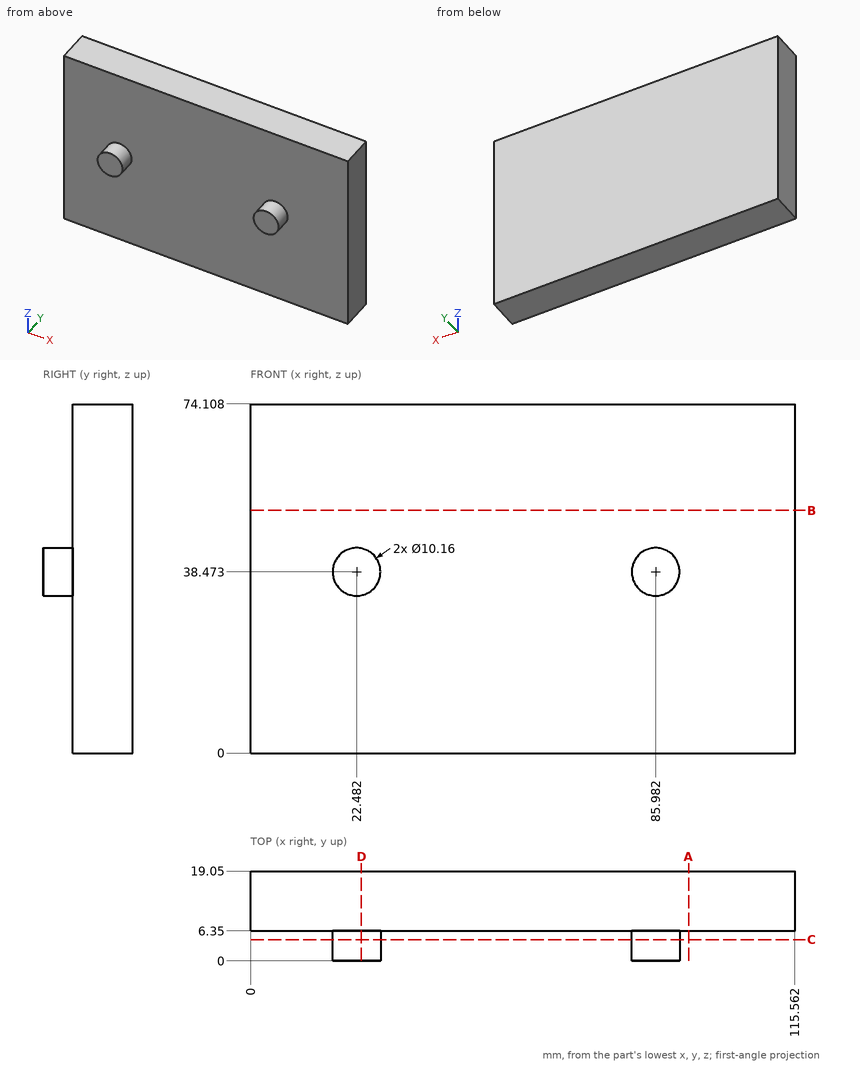
Part print with two shaded views. Sizes in mm from the minimum x, y, z corner. Coordinates: 2 decimals unless noted, no trailing zeros. Write each loop counter-clockwise with the first axis right and the second up, starting at its lowest first coordinate (ties: lowest second). Pieces come first, ordered by that corner, then holes. Notation, with made-up numbers: (63, -26.5) -> (108, -26.5) arc R17 ccw to (108, -12.5) -> close; hole circle Ø5 at (76.5, 5.5). An arc over 180 degrees is marked (long way). Return JSON: item names as keys, results as strings. Group by question number.
Q1. Cut at D-D, the plane x = 23.5. Give the cut face in (y, z), then the cut area to 3 significant figures.
Q2. Drill centre lines: line 1 (Y direction, x = 70.5, z = 14); line 2 (Z direction, x = 23, y = 5); line 3 (Z direction, x = 87.5, y = 2.75) (1 decimal). Where is each one in solid material? Low to high.
Q3. Cut at B-B, the plane z = 51.5. Give the cut face in (x, y), then the cut area to 3 significant figures.
Q4. Cut at C-C, the plane y = 4.5. Give the cut face in (x, z), then the cut area to 3 significant figures.
Q5. Flat gauge pin, fed straight in: pin 1 (1.5 mm diameter, centred on x = 102.5, z = 63.5, fed in from -Y). Where does the tip first touch, or does it go through?
Q6. Cut at A-A, the plane x = 93. Give the cut face in (y, z), then the cut area to 3 significant figures.
Returned:
{
 "1": {"outline": "(0, 33.5) -> (6.35, 33.5) -> (6.35, 0) -> (19.05, 0) -> (19.05, 74.11) -> (6.35, 74.11) -> (6.35, 43.45) -> (0, 43.45) -> close", "area": "1,000 mm2"},
 "2": {"line 1": "y = 6.35 to 19.05", "line 2": "z = 33.42 to 43.53", "line 3": "z = 33.6 to 43.3"},
 "3": {"outline": "(0, 6.35) -> (115.56, 6.35) -> (115.56, 19.05) -> (0, 19.05) -> close", "area": "1,470 mm2"},
 "4": {"outline": "circle Ø10.16 at (22.48, 38.47); circle Ø10.16 at (85.98, 38.47)", "area": "162 mm2"},
 "5": {"pin 1": "stops at y = 6.35"},
 "6": {"outline": "(6.35, 0) -> (19.05, 0) -> (19.05, 74.11) -> (6.35, 74.11) -> close", "area": "941 mm2"}
}
